Verification items for the finished model (mm, model axes). A direction names the side the tool comes from. Coordinates: 2 decimals unless noted, no trailing zeros. Write each loop counter-clockwise with the first axis right and the second up, starting at its lowest first coordinate (ties: lowest second). Pieces come first, ordered by that corner, then holes. Notation, with made-up numbers: (-37.5, 83) -> (-21.5, 83) arc R9 cw to (-21.5, 93) -> close; hole circle Ø10 at (69, 39). An arc over 180 degrees is marked (long way). Write each question's results on one line, items separated by ' | '. Start each with the question number.
from build123d import *

# Parameters (mm, degrees)
CROQUIS1_R              = 1.5
SALIENTE_EXTRUIR1_DEPTH = 2.5
SALIENTE_EXTRUIR2_START = -8.15
CROQUIS1_4_R            = 2.5
SALIENTE_EXTRUIR2_DEPTH = 7.87
SALIENTE_EXTRUIR3_DEPTH = 16.02
REDONDEO1_R             = 5
CROQUIS3_W              = 21.14
CROQUIS3_H              = 7.5
CROQUIS3_R              = 1.5
SALIENTE_EXTRUIR4_DEPTH = 2.5


with BuildPart() as part:
    # Croquis1 → Saliente-Extruir1 (new body)
    with BuildSketch(Plane(origin=(0, 0, 0), x_dir=(1, 0, 0), z_dir=(0, 1, 0))):
        Polygon((3.6, 27.14), (-3.6, 27.14), (-3.6, 12.952959179), (3.6, 6), align=None)
        with Locations(Location((-0.4, 21.14, 0), (0, 0, 270))):
            Circle(CROQUIS1_R, mode=Mode.SUBTRACT)
    extrude(amount=-SALIENTE_EXTRUIR1_DEPTH)



with BuildPart() as body_2:
    # Croquis1<4> → Saliente-Extruir2 (new body)
    with BuildSketch(Plane(origin=(0, 0, 0), x_dir=(1, 0, 0), z_dir=(0, 1, 0)).offset(SALIENTE_EXTRUIR2_START)):
        with BuildLine():
            Line((3.6, 6), (-3.6, 12.952959179))
            Line((-3.6, 12.952959179), (-3.6, 0))
            ThreePointArc((-3.6, 0), (0, -3.6), (3.6, 0))
            Line((3.6, 0), (3.6, 6))
        make_face()
        with Locations(Location((0, 0, 0), (0, 0, 270))):
            Circle(CROQUIS1_4_R, mode=Mode.SUBTRACT)
    extrude(amount=-SALIENTE_EXTRUIR2_DEPTH)


with BuildPart() as part_1:
    add(part.part)

    add(body_2.part)  # Saliente-Extruir3 merges body 2
    # Croquis1<5> → Saliente-Extruir3 (add)
    with BuildSketch(Plane(origin=(0, 0, 0), x_dir=(1, 0, 0), z_dir=(0, 1, 0))):
        Polygon((-2.286227518, 17.94), (-3.6, 17.94), (-3.6, 12.952959179), (3.6, 6), (3.6, 12.25573616), align=None)
    extrude(amount=-SALIENTE_EXTRUIR3_DEPTH)

    # Redondeo1
    redondeo1_edges = [part_1.edges().sort_by_distance(p)[0] for p in [
        (0.656886241, -16.02, -15.09786808),
    ]]
    fillet(redondeo1_edges, radius=REDONDEO1_R)

    # Croquis3 → Saliente-Extruir4 (add)
    # profile 1 of 2: a face of its own
    with BuildSketch(Plane(origin=(3.6, 0, 0), x_dir=(0, 0, -1), z_dir=(1, 0, 0))):
        with BuildLine():
            Line((6, 0), (6, -8.15))
            Line((6, -8.15), (6, -15.994937186))
            add(Edge.make_bspline(
                [(6, -15.994937186), (12.25573616, -15.542670169), (12.25573616, -11.02)],
                knots=[4.821475205, 4.821475205, 4.821475205, 6.283185307, 6.283185307, 6.283185307], degree=2, weights=[0.962144349, 0.727447175, 1]))
            Line((12.25573616, -11.02), (12.25573616, -2.5))
            Line((12.25573616, -2.5), (27.14, -2.5))
            Line((27.14, -2.5), (27.14, 0))
            Line((27.14, 0), (6, 0))
        make_face()
    # profile 2 of 2: a face of its own
    with BuildSketch(Plane(origin=(3.6, 0, 0), x_dir=(0, 0, -1), z_dir=(1, 0, 0))):
        with Locations((16.57, 3.75)):
            Rectangle(CROQUIS3_W, CROQUIS3_H)
        with Locations((11.14, 3.5)):
            Circle(CROQUIS3_R, mode=Mode.SUBTRACT)
    extrude(amount=SALIENTE_EXTRUIR4_DEPTH)


solid = part_1.part
1. Sectioned sample at C-C on x = -0.4. State how many separate pieces and enclosed holes the cut face has, plus the area to 3 significant figures.
2. Tool access check on faces 1 (the flat face through (3.6, 4, -16)), 2 (the flat face through (0.698, -6.7, -15.058)), 3 (the flat face through (5, -4, -6)). Record the directions out of +Z, -Z, +X, -X, +Y, -Y that give a thin tool (end or side, any length) a straight path to the whole face; none if there is none.
3. Depth check by flat-ended pin: pin 1 Ø3 at (x, y) = (-0.5, -12) entering from +Z; pin 2 Ø2 at (x, z) = (0.5, -1) entering from +Y; pin 3 Ø2 at (x, z) = (-1.5, -18.5) entering from +Y; pin 4 Ø0.7 at (x, y) = (5.5, -7.5) entering from -Z. Enter the tip coordinate at first touch or a pass-through.
4. Mould release check, pull along Y, two halves, no side actions. Record for faces 4 (the flat face through (2, -2.5, -21)), 5 (the flat face through (-0.05, -4.018, -9.525)), 6 (the cylindrical face through (4.83, 3.57, -9.64)): +Y half, -Y half, draft (parallel to the pull), parting line (faces both ways), or undercut.
5. Sectioned sample at B-B on y = 3.5. Record the cut outline in (x, z).
6. Sectioned sample at D-D on z = -0.5. Record the cut outline in (x, y).
7. Sectioned sample at A-A on z = -21.14. Record the cut outline in (x, y), plus the area to 3 significant figures.
8. Material ranges on probe 1 along X at (y, z) = (-12.75, 0); probe 2 along Y at (x, z) = (4.75, -16.5); probe 3 along Y at (x, z) = (2.5, -7), recorded low to high. Write a range as from..to.
Computed values:
1) separate pieces: 3 | enclosed holes: 0 | area: 180 mm^2
2) face 1: +Z, -Z, -X, +Y | face 2: -Z, +X, -Y | face 3: +Z, +X, +Y, -Y
3) pin 1: stops at z = 3.6 | pin 2: passes through | pin 3: stops at y = 0 | pin 4: stops at z = -12.26
4) face 4: -Y half | face 5: draft | face 6: undercut
5) outline: (3.6, -27.14) -> (6.1, -27.14) -> (6.1, -12.64) -> (3.6, -12.64) -> close; (3.6, -9.64) -> (6.1, -9.64) -> (6.1, -6) -> (3.6, -6) -> close
6) outline: (-3.6, -16.02) -> (-2.45, -16.02) -> (-2.45, -8.15) -> (-3.6, -8.15) -> close; (2.45, -16.02) -> (3.6, -16.02) -> (3.6, -8.15) -> (2.45, -8.15) -> close
7) outline: (-3.6, -2.5) -> (-1.9, -2.5) -> (-1.9, 0) -> (-3.6, 0) -> close; (1.1, -2.5) -> (6.1, -2.5) -> (6.1, 7.5) -> (3.6, 7.5) -> (3.6, 0) -> (1.1, 0) -> close | area: 35.5 mm^2
8) probe 1: x = -3.6..-2.5, 2.5..3.6 | probe 2: y = -2.5..7.5 | probe 3: y = -16..-8.15
